```python
from build123d import *

# Parameters (mm, degrees)
F0_R     = 100
F1_DEPTH = 18.63153
F2_R     = 4
F3_R     = 5
F4_DEPTH = 15


with BuildPart() as f1:
    # F0 (on Front) → F1 (new body)
    with BuildSketch(Plane.XZ):
        with Locations((-44.569857, 36.709767)):
            Circle(F0_R)
    extrude(amount=F1_DEPTH)

    # F2
    f2_edges = [f1.edges().sort_by_distance(p)[0] for p in [
        (-144.569857, -18.63153, 36.709767),
        (-144.569857, 0, 36.709767),
    ]]
    fillet(f2_edges, radius=F2_R)

    # F3 (on face) → F4 (join)
    with BuildSketch(Plane(origin=(0, 0, 0), x_dir=(-1, 0, 0), z_dir=(0, 1, 0))):
        with Locations((44.569857, 36.709767)):
            Circle(F3_R)
    extrude(amount=F4_DEPTH)


solid = f1.part
```
Design review of the part built by this model. Coordinates are the model's own, in mm. A direction names the side the tool comes from. Give positions to 0.01 mm unless a question says otherwise; leave off trailing zeros. Write each loop counter-clockwise with the first axis right and the second up, starting at its lowest first coordinate (ties: lowest second). Pieces come first, ordered by that corner, then holes. Notation, with made-up numbers: (-4.75, 52) - (14.25, 52) arc R30 ccw to (14.25, 83) - close; hole circle Ø10 at (-13.5, 69). An arc over 180 degrees is marked (long way). Return JSON: item names as keys, results as strings. Group by question number.
(1) We need section A-A, the plane y = -8.5. Give the boundary of the cut face in (x, z), then the cut area to 3 significant figures.
(2) To check wall thickness, follow probe 1 along Y at (x, z) = (-43, -35); probe 2 along Z at (x, y) = (-47.5, -10.5); probe 3 along X at (y, z) = (-5.5, 34). State the ranges of each line that lie inside material, in increasing order.
(3) Insertion check: pin 1 (3 mm diameter, centred on x = -57, z = 96, fed in from +Y); pin 2 (3 mm diameter, centred on x = -47.5, y = -7.5, fed in from -Z); pin 3 (8 mm diameter, centred on y = -10, z = -21.5, fed in from +X). Each pin has a flat end and moves straight along its axis. Give the tip position at first contact, or say it passes through.
(4) We need section B-B, the plane y = 3.5. Give the boundary of the cut face in (x, z), then the cut area to 3 significant figures.
(5) Machinability: for faces 1 (the flat face through (-44, 15, 37)), 2 (the cylindrical face through (-49.34, 7.4, 38.21)), which of the approach directions +Z, -Z, +X, -X, +Y, -Y give a long, thin tool a straight path to every point of the face, cutting with its end or side? Answer none if there is none.
Reported:
{
 "1": {"outline": "circle Ø200 at (-44.57, 36.71)", "area": "31,400 mm2"},
 "2": {"probe 1": "y = -18.63 to 0", "probe 2": "z = -63.25 to 136.67", "probe 3": "x = -144.53 to 55.39"},
 "3": {"pin 1": "stops at y = 0", "pin 2": "stops at z = -63.28", "pin 3": "stops at x = 39.46"},
 "4": {"outline": "circle Ø10 at (-44.57, 36.71)", "area": "78.5 mm2"},
 "5": {"face 1": "+Z, -Z, +X, -X, +Y", "face 2": "+Y"}
}
